from build123d import *

# Parameters (mm, degrees)
BOSS_EXTRUDE1_REACH      = 78.759
BOSS_EXTRUDE1_END_RADIUS = 22
SKETCH2_R                = 4
SKETCH2_R_2              = 3
SKETCH3_R                = 3
CUT_EXTRUDE1_DEPTH       = 77.75936425


with BuildPart() as part:
    # Sketch1 → Revolve1 (revolve)
    with BuildSketch(Plane.XY, mode=Mode.PRIVATE) as revolve1_sk:
        Polygon((-32, 18), (-32, 32), (-23, 32), (-23, 24), (-14, 24), (-14, 22), (14, 22), (14, 24), (23, 24), (23, 32), (32, 32), (32, 18), align=None)
    revolve(revolve1_sk.sketch.rotate(Axis((-55.697732997, 0, 0), (1, 0, 0)), 90), axis=Axis((-55.697732997, 0, 0), (1, 0, 0)))

    # Boss-Extrude1: up to this cylinder (the profile starts outside it)
    boss_extrude1_end = Plane(origin=(0, 0, 0), z_dir=(-1, 0, 0)) * Cylinder(BOSS_EXTRUDE1_END_RADIUS, 202.518, mode=Mode.PRIVATE)
    # Sketch2 → Boss-Extrude1 (add, up to the surface)
    with BuildSketch(Plane(origin=(0, -30, 0), x_dir=(1, 0, 0), z_dir=(0, 1, 0)), mode=Mode.PRIVATE) as boss_extrude1_sk1:
        with Locations(Location((0, 0, 0), (0, 0, 90))):
            Circle(SKETCH2_R)
        with Locations(Location((0, 0, 0), (0, 0, 90))):
            Circle(SKETCH2_R_2, mode=Mode.SUBTRACT)
    boss_extrude1_tool1 = extrude(boss_extrude1_sk1.sketch, amount=BOSS_EXTRUDE1_REACH, mode=Mode.PRIVATE) - boss_extrude1_end
    add(boss_extrude1_tool1.solids().sort_by_distance((0, -30, 3.886863))[0])

    # Sketch3 → Cut-Extrude1 (cut, through all)
    with BuildSketch(Plane.XZ.offset(30)):
        with Locations(Location((0, 0, 0), (0, 0, 270))):
            Circle(SKETCH3_R)
    extrude(amount=-CUT_EXTRUDE1_DEPTH, mode=Mode.SUBTRACT)


solid = part.part
Geometry check sheet. Reference: the model listing, model coordinates, mm. A direction names the side the tool comes from. Give positions to 0.01 mm unless a question says otherwise; leave off trailing zeros. Write each loop counter-clockwise with the first axis right and the second up, starting at its lowest first coordinate (ties: lowest second). Pieces come first, ordered by that corner, then holes. Notation, with made-up numbers: M 18.5,63 L 42.5,63 A12 cw 42.5,74 Z; hole C 55.25,-14.75 d10. An arc over 180 degrees is marked long. Answer as CSV lines item,"result". Start each with the question number.
Q1. Section check D-D, the plane x = 27.5. Record the cut outline in (y, z).
Q2. Section check A-A, the plane y = 0. Record the cut outline in (x, z), then the cut area to 3 significant figures.
Q3. Tool access check on faces 5 (the face through (-3, -30, -1)), 6 (the face through (3.905, -25.875, 0.867)), 7 (the face through (0.196, 21.477, -4.769)). Record the directions out of +Z, -Z, +X, -X, +Y, -Y that give a thin tool (end or side, any length) a straight path to the whole face; none if there is none.
Q4. Section check B-B, the plane z = -16. Record the cut outline in (x, y), then the cut area to 3 significant figures.
Q5. Release check for a two-part mould opening along Z. For faces 1 (the face through (-14, 21.2, 7)), 2 (the face through (0.9, 19.85, -2.86)), 3 (the face through (-27.44, 31.24, -6.94)), 4 (the face through (-0.448, 17.572, -3.902)) record: pulls with the +Z half, pulls with the -Z half, needs draft (parallel to the pull), parting line crosses it, or undercut.
Q6. Go/stop test with flat-tipped pins: pin 1 (2 mm diameter, centred on x = -9, y = 5, fed in from +Z); pin 2 (5.5 mm diameter, centred on x = 0, z = 0, fed in from +Y); pin 3 (1.5 mm diameter, centred on x = -5, y = -10.5, fed in from +Z); pin 4 (12 mm diameter, centred on x = 20.5, z = -5, fed in from -Y). Record where each tip stops, or that it passes through.
Q7. Material ranges on L1, parallel to X at y = -25, z = 0; L2, parallel to X at y = -14, z = 18; L3, parallel to X at y = 20.9, z = 0, recorded low to high.
Q8. Section check C-C, the plane x = 0. Record the cut outline in (y, z).
Geometry says:
1,outline,"C 0,0 d64; hole C 0,0 d36"
2,outline,"M -32,-32 L -23,-32 L -23,-24 L -14,-24 L -14,-22 L 14,-22 L 14,-24 L 23,-24 L 23,-32 L 32,-32 L 32,-18 L -32,-18 Z; M -32,18 L 32,18 L 32,32 L 23,32 L 23,24 L 14,24 L 14,22 L -14,22 L -14,24 L -23,24 L -23,32 L -32,32 Z"
2,area,"944 mm^2"
3,face 5,"+Z, -Z, -Y"
3,face 6,"-Y"
3,face 7,"none"
4,outline,"M -32,-27.71 L -23,-27.71 L -23,-17.89 L -14,-17.89 L -14,-15.1 L 14,-15.1 L 14,-17.89 L 23,-17.89 L 23,-27.71 L 32,-27.71 L 32,-8.25 L -32,-8.25 Z; M -32,8.25 L 32,8.25 L 32,27.71 L 23,27.71 L 23,17.89 L 14,17.89 L 14,15.1 L -14,15.1 L -14,17.89 L -23,17.89 L -23,27.71 L -32,27.71 Z"
4,area,"1,430 mm^2"
5,face 1,"needs draft"
5,face 2,"undercut"
5,face 3,"parting line crosses it"
5,face 4,"undercut"
6,pin 1,"z = 21.63"
6,pin 2,"through"
6,pin 3,"z = 19.72"
6,pin 4,"y = -32"
7,L1,"-32 to -23, -4 to -3, 3 to 4, 23 to 32"
7,L2,"-32 to -14, 14 to 32"
7,L3,"-32 to -3, 3 to 32"
8,outline,"M -30,-4 L -21.63,-4 A22 ccw 21.79,-3 L 17.75,-3 A18 cw -17.75,-3 L -30,-3 Z; M -30,3 L -17.75,3 A18 cw 17.75,3 L 21.79,3 A22 ccw -21.63,4 L -30,4 Z"
